from build123d import *

# Parameters (mm, degrees)
F1_DEPTH = 100
F2_R     = 4
F3_DEPTH = 25


with BuildPart() as f1:
    # F0 (on Front) → F1 (new body)
    with BuildSketch(Plane.XZ):
        Polygon((-6.551726, 42.5), (-19.051726, 42.5), (-19.051726, 0), (-19.051726, -42.5), (-6.551726, -42.5), (-6.551726, -39.5), (-9.551726, -39.5), (-9.551726, -20), (-13.051726, -20), (-13.051726, 0), (-13.051726, 20), (-9.551726, 20), (-9.551726, 39.5), (-6.551726, 39.5), align=None)
    extrude(amount=F1_DEPTH)

    # F2 (on face) → F3 (cut)
    with BuildSketch(Plane(origin=(-19.051726, 0, 0), x_dir=(0, -1, 0), z_dir=(-1, 0, 0))):
        with Locations((25, 25)):
            Circle(F2_R)
        with Locations((75, 25)):
            Circle(F2_R)
        with Locations((25, -25)):
            Circle(F2_R)
        with Locations((75, -25)):
            Circle(F2_R)
    extrude(amount=-F3_DEPTH, mode=Mode.SUBTRACT)


solid = f1.part
Here's how the part is built. I have some questions about the finished solid (model axes, mm). A direction names the side the tool comes from. Round coordinates to 2 decimals unless told otherwise and drop trailing zeros. Loops run counter-clockwise (first coordinate to the right, second up) from the corner with the lowest first, then second, coordinate; pieces in that order, holes last. Notation, with made-up numbers: M 66,54 L 71,54 A14 ccw 71,67 Z; hole C -3,-36 d3. An arc over 180 degrees is marked long. Write each question's results on one line, items separated by ' | '. Start each with the question number.
(1) I want a section at A-A (y = -25). Please give me the cut outline in (x, z).
(2) I want a section at C-C (z = -25). Please give me the cut outline in (x, y).
(3) On a 3-axis mill with a long thin cutter (end or side, diameter ignored), from which of +Z, -Z, +X, -X, +Y, -Y can I reach the whole of each face in a straight line? I mean faces 1 (the flat face through (-8, -49, -39.5)), 2 (the cylindrical face through (-14.368, -24.479, 28.966)). Say none if no direction works.
(4) Will these pins go through, and if not, where does the flat tip stop? P1, Ø6, axis at y = -69.5, z = 32.5, coming from the +X side; P2, Ø4, axis at x = -9, z = -26, coming from the -Y side; P3, Ø12, axis at y = -37, z = 4, coming from the +X side.
(5) I want a section at B-B (x = -16). Please give me the cut outline in (y, z).
(6) If I drill on probe 1 along Z at (x, y) = (-14.5, -75); probe 2 along Z at (x, y) = (-9.25, -77); probe 3 along Y at (x, z) = (-10, 22), over which ranges is the centre line in solid material (lowest first)? Write a range as from..to.
(7) I want a section at D-D (y = -89). Please give me the cut outline in (x, z), then the cut area to 4 significant figures.
(8) Thinking about a two-plate mould opening in Y: for faces 3 (the cylindrical face through (-14.368, -74.479, 28.966)), 4 (the flat face through (-9.552, -49, 30)), 5 (the flat face through (-16, -100, 1)), which applies, pulls with the +Y half, pulls with the -Y half, needs draft (parallel to the pull), parting line crosses it, or undercut?
Solved:
1) outline: M -19.05,-42.5 L -6.55,-42.5 L -6.55,-39.5 L -9.55,-39.5 L -9.55,-29 L -19.05,-29 Z; M -19.05,-21 L -9.55,-21 L -9.55,-20 L -13.05,-20 L -13.05,20 L -9.55,20 L -9.55,21 L -19.05,21 Z; M -19.05,29 L -9.55,29 L -9.55,39.5 L -6.55,39.5 L -6.55,42.5 L -19.05,42.5 Z
2) outline: M -19.05,-100 L -9.55,-100 L -9.55,-79 L -19.05,-79 Z; M -19.05,-71 L -9.55,-71 L -9.55,-29 L -19.05,-29 Z; M -19.05,-21 L -9.55,-21 L -9.55,0 L -19.05,0 Z
3) face 1: +X, +Y, -Y | face 2: +X, -X
4) P1: stops at x = -9.55 | P2: stops at y = -100 | P3: stops at x = -13.05
5) outline: M -100,-42.5 L 0,-42.5 L 0,42.5 L -100,42.5 Z; hole C -75,-25 d8; hole C -75,25 d8; hole C -25,-25 d8; hole C -25,25 d8
6) probe 1: z = -42.5..-29, -21..21, 29..42.5 | probe 2: z = -42.5..-39.5, 39.5..42.5 | probe 3: y = -100..-77.65, -72.35..-27.65, -22.35..0
7) outline: M -19.05,-42.5 L -6.55,-42.5 L -6.55,-39.5 L -9.55,-39.5 L -9.55,-20 L -13.05,-20 L -13.05,20 L -9.55,20 L -9.55,39.5 L -6.55,39.5 L -6.55,42.5 L -19.05,42.5 Z | area: 685.5 mm²
8) face 3: undercut | face 4: needs draft | face 5: pulls with the -Y half
